```python
from build123d import *

# Parameters (mm, degrees)
F0_W     = 91
F0_H     = 64
F1_DEPTH = 40
F2_W     = 89.5
F2_H     = 62.5
F3_DEPTH = 39
F4_R     = 5
F5_R     = 2.5


with BuildPart() as f1:
    # F0 (on Top) → F1 (new body)
    with BuildSketch(Plane.XY):
        Rectangle(F0_W, F0_H)
    extrude(amount=F1_DEPTH)

    # F2 (on face) → F3 (cut)
    with BuildSketch(Plane.XY.offset(40)):
        Rectangle(F2_W, F2_H)
    extrude(amount=-F3_DEPTH, mode=Mode.SUBTRACT)

    # F4
    f4_edges = [f1.edges().sort_by_distance(p)[0] for p in [
        (0, 31.25, 1),
        (-44.75, 0, 1),
        (0, -31.25, 1),
        (44.75, 0, 1),
    ]]
    fillet(f4_edges, radius=F4_R)

    # F5
    f5_edges = [f1.edges().sort_by_distance(p)[0] for p in [
        (45.5, 0, 0),
        (0, 32, 0),
        (-45.5, 0, 0),
        (0, -32, 0),
    ]]
    fillet(f5_edges, radius=F5_R)


solid = f1.part
```
Part model, mm, in its own coordinate system. A direction names the side the tool comes from. Round coordinates to 2 decimals unless told otherwise and drop trailing zeros. Order: outer loops, then holes, each group sorted by start corner. A loop starts at its lowest first (then second) coordinate and runs counter-clockwise, first axis right, second up. Notation, with made-up numbers: M 16.25,38.25 L 66.25,38.25 A28 cw 66.25,66.25 Z; hole C 3,76.25 d11. An arc over 180 degrees is marked long. Answer in a Markdown table with one row per item. Add a question column.
Q1. Cut at C-C on y = 9.5. Give the cut face in (x, z).
Q2. Mould opens along Y. For faces 1 (the face through (-45, 0, 1)), 2 (the face through (-1, 32, 21)), 3 (the face through (-1, -32, 21)), 4 (the face through (-1, 0, 1)) say: +Y half, -Y half, draft (parallel to the pull), parting line (faces both ways), or undercut.
Q3. Pin check, flat tip, straight feed: pin 1 (12 mm diameter, centred on x = -28, y = 18, fed in from +Z). Stop position of the tip, or through.
Q4. Wall check: L1, parallel to X at y = 11.5, z = 27; L2, parallel to Y at x = -8, z = 33; L3, parallel to Z at x = -32, y = -25. Give the ranges that are in metal, low to high. Write a range as from..to.
Q5. Cut at B-B on x = 29. Give the cut face in (y, z), and give its area (3 significant figures).
Q6. 3-axis set-ups, long thin cutter, end or side, ignore diameter. For faces 5 (the face through (-1, 0, 0)), 6 (the face through (0.63, -29.82, 2.5)): which of +Z, -Z, +X, -X, +Y, -Y reach the whole face in a straight line?
Q7. Cut at A-A on z = 20.5. Give the cut face in (x, y).
Established:
| question | item | result |
|---|---|---|
| 1 | outline | M -45.5,2.5 A2.5 ccw -43,0 L 43,0 A2.5 ccw 45.5,2.5 L 45.5,40 L 44.75,40 L 44.75,6 A5 cw 39.75,1 L -39.75,1 A5 cw -44.75,6 L -44.75,40 L -45.5,40 Z |
| 2 | face 1 | draft |
| 2 | face 2 | +Y half |
| 2 | face 3 | -Y half |
| 2 | face 4 | undercut |
| 3 | pin 1 | stops at z = 1 |
| 4 | L1 | x = -45.5..-44.75, 44.75..45.5 |
| 4 | L2 | y = -32..-31.25, 31.25..32 |
| 4 | L3 | z = 0..1 |
| 5 | outline | M -32,2.5 A2.5 ccw -29.5,0 L 29.5,0 A2.5 ccw 32,2.5 L 32,40 L 31.25,40 L 31.25,6 A5 cw 26.25,1 L -26.25,1 A5 cw -31.25,6 L -31.25,40 L -32,40 Z |
| 5 | area | 131 mm2 |
| 6 | face 5 | -Z, +X, -X, +Y, -Y |
| 6 | face 6 | +Z |
| 7 | outline | M -45.5,-32 L 45.5,-32 L 45.5,32 L -45.5,32 Z; hole M -44.75,-31.25 L 44.75,-31.25 L 44.75,31.25 L -44.75,31.25 Z |
